```python
from build123d import *

# Parameters (mm, degrees)
F0_W     = 180
F0_H     = 10
F0_R     = 0.5
F1_DEPTH = 2
F2_R     = 4.99999


# Not quite as in the source:
# - a fillet or chamfer is up to 0.001 mm smaller than in the source, because OpenCascade refuses the exact size


with BuildPart() as f1:
    # F0 (on Right) → F1 (new body)
    with BuildSketch(Plane.YZ):
        Polygon((78.3572724922, 47.473322805), (78.3572724922, 12.473322805), (78.3572724922, 2.473322805), (78.3572724922, -12.526677195), (93.3572724922, -12.526677195), (93.3572724922, 47.473322805), align=None)
        with Locations((-11.6427275078, 7.473322805)):
            Rectangle(F0_W, F0_H)
        with Locations((-96.7759713531, 7.473322805)):
            Circle(F0_R, mode=Mode.SUBTRACT)
        with Locations((-94.7759713531, 7.473322805)):
            Circle(F0_R, mode=Mode.SUBTRACT)
        with Locations((-92.7759713531, 7.473322805)):
            Circle(F0_R, mode=Mode.SUBTRACT)
        with Locations((-90.7759713531, 7.473322805)):
            Circle(F0_R, mode=Mode.SUBTRACT)
        with Locations((-88.7759713531, 7.473322805)):
            Circle(F0_R, mode=Mode.SUBTRACT)
        with Locations((-86.7759713531, 7.473322805)):
            Circle(F0_R, mode=Mode.SUBTRACT)
        with Locations((-84.7759713531, 7.473322805)):
            Circle(F0_R, mode=Mode.SUBTRACT)
        with Locations((-82.7759713531, 7.473322805)):
            Circle(F0_R, mode=Mode.SUBTRACT)
        with Locations((-80.7759713531, 7.473322805)):
            Circle(F0_R, mode=Mode.SUBTRACT)
        with Locations((-78.7759713531, 7.473322805)):
            Circle(F0_R, mode=Mode.SUBTRACT)
        with Locations((-76.7759713531, 7.473322805)):
            Circle(F0_R, mode=Mode.SUBTRACT)
        with Locations((-74.7759713531, 7.473322805)):
            Circle(F0_R, mode=Mode.SUBTRACT)
        with Locations((-72.7759713531, 7.473322805)):
            Circle(F0_R, mode=Mode.SUBTRACT)
        with Locations((-70.7759713531, 7.473322805)):
            Circle(F0_R, mode=Mode.SUBTRACT)
        with Locations((-68.7759713531, 7.473322805)):
            Circle(F0_R, mode=Mode.SUBTRACT)
        with Locations((-66.7759713531, 7.473322805)):
            Circle(F0_R, mode=Mode.SUBTRACT)
        with Locations((-64.7759713531, 7.473322805)):
            Circle(F0_R, mode=Mode.SUBTRACT)
        with Locations((-62.7759713531, 7.473322805)):
            Circle(F0_R, mode=Mode.SUBTRACT)
        with Locations((-60.7759713531, 7.473322805)):
            Circle(F0_R, mode=Mode.SUBTRACT)
        with Locations((-58.7759713531, 7.473322805)):
            Circle(F0_R, mode=Mode.SUBTRACT)
        with Locations((-56.7759713531, 7.473322805)):
            Circle(F0_R, mode=Mode.SUBTRACT)
        with Locations((-54.7759713531, 7.473322805)):
            Circle(F0_R, mode=Mode.SUBTRACT)
        with Locations((-52.7759713531, 7.473322805)):
            Circle(F0_R, mode=Mode.SUBTRACT)
        with Locations((-50.7759713531, 7.473322805)):
            Circle(F0_R, mode=Mode.SUBTRACT)
        with Locations((-48.7759713531, 7.473322805)):
            Circle(F0_R, mode=Mode.SUBTRACT)
        with Locations((-46.7759713531, 7.473322805)):
            Circle(F0_R, mode=Mode.SUBTRACT)
        with Locations((-44.7759713531, 7.473322805)):
            Circle(F0_R, mode=Mode.SUBTRACT)
        with Locations((-42.7759713531, 7.473322805)):
            Circle(F0_R, mode=Mode.SUBTRACT)
        with Locations((-40.7759713531, 7.473322805)):
            Circle(F0_R, mode=Mode.SUBTRACT)
        with Locations((-38.7759713531, 7.473322805)):
            Circle(F0_R, mode=Mode.SUBTRACT)
        with Locations((-36.7759713531, 7.473322805)):
            Circle(F0_R, mode=Mode.SUBTRACT)
        with Locations((-34.7759713531, 7.473322805)):
            Circle(F0_R, mode=Mode.SUBTRACT)
        with Locations((-32.7759713531, 7.473322805)):
            Circle(F0_R, mode=Mode.SUBTRACT)
        with Locations((-30.7759713531, 7.473322805)):
            Circle(F0_R, mode=Mode.SUBTRACT)
        with Locations((-28.7759713531, 7.473322805)):
            Circle(F0_R, mode=Mode.SUBTRACT)
        with Locations((-26.7759713531, 7.473322805)):
            Circle(F0_R, mode=Mode.SUBTRACT)
        with Locations((-24.7759713531, 7.473322805)):
            Circle(F0_R, mode=Mode.SUBTRACT)
        with Locations((-22.7759713531, 7.473322805)):
            Circle(F0_R, mode=Mode.SUBTRACT)
        with Locations((-20.7759713531, 7.473322805)):
            Circle(F0_R, mode=Mode.SUBTRACT)
        with Locations((-18.7759713531, 7.473322805)):
            Circle(F0_R, mode=Mode.SUBTRACT)
        with Locations((-16.7759713531, 7.473322805)):
            Circle(F0_R, mode=Mode.SUBTRACT)
        with Locations((-14.7759713531, 7.473322805)):
            Circle(F0_R, mode=Mode.SUBTRACT)
        with Locations((-12.7759713531, 7.473322805)):
            Circle(F0_R, mode=Mode.SUBTRACT)
        with Locations((-10.7759713531, 7.473322805)):
            Circle(F0_R, mode=Mode.SUBTRACT)
        with Locations((-8.7759713531, 7.473322805)):
            Circle(F0_R, mode=Mode.SUBTRACT)
        with Locations((-6.7759713531, 7.473322805)):
            Circle(F0_R, mode=Mode.SUBTRACT)
        with Locations((-4.7759713531, 7.473322805)):
            Circle(F0_R, mode=Mode.SUBTRACT)
        with Locations((-2.7759713531, 7.473322805)):
            Circle(F0_R, mode=Mode.SUBTRACT)
        with Locations((-0.7759713531, 7.473322805)):
            Circle(F0_R, mode=Mode.SUBTRACT)
        with Locations((1.2240286469, 7.473322805)):
            Circle(F0_R, mode=Mode.SUBTRACT)
        Polygon((93.3572724922, -12.526677195), (78.3572724922, -12.526677195), (85.8572724922, -41.5740522915), align=None)
    extrude(amount=F1_DEPTH)

    # F2 (radius 5 in the source; OpenCascade refuses exactly that, so slightly less here)
    f2_edges = [f1.edges().sort_by_distance(p)[0] for p in [
        (1, 93.357272, 47.473323),
        (1, 78.357272, 47.473323),
        (1, 78.357272, 12.473323),
        (1, 78.357272, 2.473323),
        (1, 78.357272, -12.526677),
        (1, 93.357272, -12.526677),
        (1, -101.642728, 12.473323),
        (1, -101.642728, 2.473323),
    ]]
    fillet(f2_edges, radius=F2_R)


solid = f1.part
```
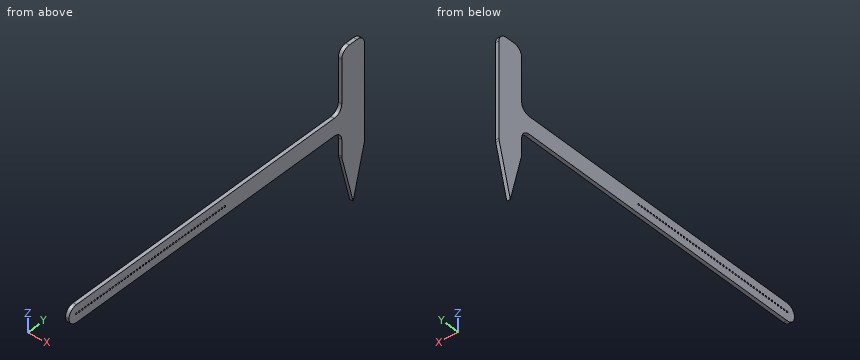
Read the model definition and answer for the solid it produces. Units are mm, in the model's axes. Coordinates: 2 decimals unless noted, no trailing zeros. Write each loop counter-clockwise with the first axis right and the second up, starting at its lowest first coordinate (ties: lowest second). Pieces come first, ordered by that corner, then holes. Notation, with made-up numbers: (12.25, -22.75) -> (17.25, -22.75) arc R12 ccw to (17.25, -7.75) -> close; hole circle Ø9 at (10, 63.25). An arc over 180 degrees is marked (long way). Write item = value, one per line.
(1) Section C-C on z = 0 is taken. Write down the section's boundary in (x, y).
From the geometry:
outline = (0, 77.67) -> (2, 77.67) -> (2, 93.36) -> (0, 93.36) -> close
(2) Given pin 1 Ø1 at (x, z) = (0.5, 27) entering from -Y; pin 2 Ø0.6 at (x, y) = (1, 20.5) entering from +Z, each flat-ended and moving along its own axis, determine where each tip first touches the part or whether it passes through.
From the geometry:
pin_1 = 78.36
pin_2 = 12.47
(3) Section A-A on x = 1.55 is taken. Count the separate pieces of the cut face and the enclosed holes in it, plus the area to 3 significant figures.
From the geometry:
separate_pieces = 1
enclosed_holes = 50
area = 2,870 mm2
(4) Straight lines are drawn through the part: L1, parallel to Y at x = 0.25, z = 21.5; L2, parallel to Z at x = 0.55, y = -70; L3, parallel to Z at x = 1.1, y = -45. For each, find the intervals that lie inside material, in ascending order. Write a range as from..to.
From the geometry:
L1 = 78.36..93.36
L2 = 2.47..12.47
L3 = 2.47..7.03, 7.92..12.47
(5) Section B-B on y = 40.5 is taken. Write down the section's boundary in (x, z), plus the area to 3 significant figures.
From the geometry:
outline = (0, 2.47) -> (2, 2.47) -> (2, 12.47) -> (0, 12.47) -> close
area = 20.0 mm2
